Autodesk Inventor part; units mm, degrees
ref_plane "ip_cst_1_or_1_XY" through (0, 0, 0) normal (1, 0, 0) x (0, 0, -1)
ref_plane "ip_cst_1_or_1_YZ" through (0, 0, 0) normal (0, 0, -1) x (0, 1, 0)
ref_plane "ip_cst_1_or_1_ZX" through (0, 0, 0) normal (0, 1, 0) x (1, 0, 0)
sketch "Sketch_1" plane through (0, 0, 0) normal (0, 0, 1) x (1, 0, 0)
  line L0 (14, 0) -> (0, 0)
  line L1 (0, 28) -> (0.644, 28)
  line L2 (0.644, 28) -> (0.644, 27.05)
  line L3 (0.644, 27.05) -> (5.1157, 27.05)
  arc A0 (8.8843, 27.05) -> (5.1157, 27.05) centre (7, 24.25) ccw
  line L4 (8.8843, 27.05) -> (13.356, 27.05)
  line L5 (13.356, 27.05) -> (13.356, 28)
  line L6 (13.356, 28) -> (14, 28)
  line L7 (14, 28) -> (14, 30)
  arc A1 (14, 30) -> (13, 31) centre (13, 30) ccw
  line L8 (13, 31) -> (1, 31)
  arc A2 (1, 31) -> (0, 30) centre (1, 30) ccw
  line L9 (0, 30) -> (0, 28)
revolve "Revolution1" add sketch "Sketch_1" angle 360 about axis through (14, 0, 0) along (1, 0, 0)
ref_plane "ip_cst_1_or_1_XY" through (0, 0, 0) normal (1, 0, 0) x (0, 0, -1)
ref_plane "ip_cst_1_or_1_YZ" through (0, 0, 0) normal (0, 0, -1) x (0, 1, 0)
ref_plane "ip_cst_1_or_1_ZX" through (0, 0, 0) normal (0, 1, 0) x (1, 0, 0)
ref_plane "ip_cst_1_or_2_XY" through (0, 0, 0) normal (-1, 0, 0) x (0, 0, -1)
ref_plane "ip_cst_1_or_2_YZ" through (0, 0, 0) normal (0, 0, -1) x (0, -1, 0)
ref_plane "ip_cst_1_or_2_ZX" through (0, 0, 0) normal (0, -1, 0) x (-1, 0, 0)
ref_plane "ip_cst_1_or_3_XY" through (0.644, 0, 0) normal (1, 0, 0) x (0, 0, -1)
ref_plane "ip_cst_1_or_3_YZ" through (0.644, 0, 0) normal (0, 0, -1) x (0, 1, 0)
ref_plane "ip_cst_1_or_3_ZX" through (0.644, 0, 0) normal (0, 1, 0) x (1, 0, 0)
ref_plane "ip_cst_1_or_4_XY" through (13.356, 0, 0) normal (-1, 0, 0) x (0, 0, -1)
ref_plane "ip_cst_1_or_4_YZ" through (13.356, 0, 0) normal (0, 0, -1) x (0, -1, 0)
ref_plane "ip_cst_1_or_4_ZX" through (13.356, 0, 0) normal (0, -1, 0) x (-1, 0, 0)
properties part number "6007DDU Outer ring"
Can you work these out from the model? Positions are in its coordinate system, mm. A direction names the side the tool comes from. Coordinates: 2 decimals unless noted, no trailing zeros. Loops run counter-clockwise (first coordinate to the right, second up) from the corner with the lowest first, then second, coordinate; pieces in that order, holes last. Notation, with made-up numbers: (54.5, -11) -> (58.5, -11) arc R19 cw to (58.5, 8) -> close; hole circle Ø11 at (31.5, 18.25). An arc over 180 degrees is marked (long way). Put each result on its own line as item: value. Start each with the question number.
Q1. I want a section at D-D (x = 6). Write out the boundary of the cut face in (y, z), plus the area to 3 significant figures.
Q2. If I drill on line 1 (Z direction, x = 3.6, y = 0); line 2 (Y direction, x = 11.25, z = -22.5); line 3 (Z direction, x = 0.2, y = 0), over which ranges is the centre line in solid material (lowest first)? Write a range as [from, to].
Q3. I want a section at C-C (x = 10.75). Write out the boundary of the cut face in (y, z).
Q4. For faces 4 (the face through (0.327, 25.865, -10.724)), 5 (the face through (2.911, -21.466, -16.46)), 6 (the face through (13.356, -15, 23)), which set-ups out of +Z, -Z, +X, -X, +Y, -Y let a thin tool reach every point of the face, with its end or its side?
Q5. Thinking about a two-plate mould opening in Z: for faces 1 (the face through (0.644, -15, 23)), 2 (the face through (14, -25, 13)), 3 (the face through (6.916, -4.036, -30.736)), which applies, pulls with the +Z half, pulls with the -Z half, needs draft (parallel to the pull), parting line crosses it, or undercut?
Q6. I'm going to push flat-ended pins straight in: P1, Ø1.5, axis at x = 3, z = -10.5, coming from the +Y side; P2, Ø1.5, axis at x = 9, z = -14, coming from the -Y side; P3, Ø1, axis at x = 8.5, y = -15, coming from the -Z side; P4, Ø3, axis at y = -23, z = -16.5, coming from the -X side. Where does each tip first touch, or does it pass through?
Q7. I want a section at A-A (y = 0). Write out the boundary of the cut face in (x, z) (3 decimals), plus the area to 3 significant figures.
Taken from the geometry:
1. outline: circle Ø62 at (0, 0); hole circle Ø54.95 at (0, 0)
1. area: 648 mm2
2. line 1: z = [-31, -27.05], [27.05, 31]
2. line 2: y = [-21.32, -15.02], [15.02, 21.32]
2. line 3: z = [-30.6, -28], [28, 30.6]
3. outline: circle Ø62 at (0, 0); hole circle Ø54.1 at (0, 0)
4. face 4: -X
4. face 5: +X, -X
4. face 6: +X
5. face 1: undercut
5. face 2: needs draft
5. face 3: parting line crosses it
6. P1: stops at y = 29.43
6. P2: stops at y = -28.03
6. P3: stops at z = -27.4
6. P4: stops at x = 0
7. outline: (0, -30) arc R1 ccw to (1, -31) -> (13, -31) arc R1 ccw to (14, -30) -> (14, -28) -> (13.356, -28) -> (13.356, -27.05) -> (8.884, -27.05) arc R3.375 cw to (5.116, -27.05) -> (0.644, -27.05) -> (0.644, -28) -> (0, -28) -> close; (0, 28) -> (0.644, 28) -> (0.644, 27.05) -> (5.116, 27.05) arc R3.375 cw to (8.884, 27.05) -> (13.356, 27.05) -> (13.356, 28) -> (14, 28) -> (14, 30) arc R1 ccw to (13, 31) -> (1, 31) arc R1 ccw to (0, 30) -> close
7. area: 104 mm2
